Work out the finished part from the listing and answer in its coordinate system (mm). A direction names the side the tool comes from. Give positions to 0.01 mm unless a question says otherwise; leave off trailing zeros. Loops run counter-clockwise (first coordinate to the right, second up) from the corner with the lowest first, then second, coordinate; pieces in that order, holes last. Notation, with made-up numbers: (50.5, 44) - (90.5, 44) arc R20 cw to (90.5, 61) - close; hole circle Ø8 at (8, 26.5). An arc over 180 degrees is marked (long way). One line per question, with ' | ' between items.
from build123d import *

# Parameters (mm, degrees)
F0_R     = 1.7272
F0_R_2   = 2.15265
F0_R_3   = 9.525
F0_R_4   = 36.195
F1_DEPTH = 3.175
F2_R     = 4.7625


with BuildPart() as f1:
    # F0 (on Top) → F1 (new body)
    with BuildSketch(Plane.XY):
        with BuildLine():
            Line((-19.1686927371, 36.195), (-66.6623, 36.195))
            Line((-66.6623, 36.195), (-66.6623, -35.3695))
            Line((-66.6623, -35.3695), (-44.2988323935, -35.3695))
            Line((-44.2988323935, -35.3695), (-14.5929161967, -65.0754161967))
            ThreePointArc((-14.5929161967, -65.0754161967), (0, -71.12), (14.5929161967, -65.0754161967))
            Line((14.5929161967, -65.0754161967), (44.2988323935, -35.3695))
            Line((44.2988323935, -35.3695), (66.6623, -35.3695))
            Line((66.6623, -35.3695), (66.6623, 36.195))
            Line((66.6623, 36.195), (19.1686927371, 36.195))
            ThreePointArc((19.1686927371, 36.195), (0, 40.9575), (-19.1686927371, 36.195))
        make_face()
        with Locations((-11.7865861589, -62.2690861589)):
            Circle(F0_R, mode=Mode.SUBTRACT)
        with Locations((-61.8998, -30.607)):
            Circle(F0_R_2, mode=Mode.SUBTRACT)
        with Locations((-11.7865861589, -38.6959138411)):
            Circle(F0_R, mode=Mode.SUBTRACT)
        with Locations((11.7865861589, -62.2690861589)):
            Circle(F0_R, mode=Mode.SUBTRACT)
        with Locations((0, -50.4825)):
            Circle(F0_R_3, mode=Mode.SUBTRACT)
        with Locations((11.7865861589, -38.6959138411)):
            Circle(F0_R, mode=Mode.SUBTRACT)
        with Locations((61.8998, -30.607)):
            Circle(F0_R_2, mode=Mode.SUBTRACT)
        with Locations((-61.8998, 31.4325)):
            Circle(F0_R_2, mode=Mode.SUBTRACT)
        Circle(F0_R_4, mode=Mode.SUBTRACT)
        with Locations((61.8998, 31.4325)):
            Circle(F0_R_2, mode=Mode.SUBTRACT)
    extrude(amount=F1_DEPTH)

    # F2
    f2_edges = [f1.edges().sort_by_distance(p)[0] for p in [
        (66.6623, -35.3695, 1.5875),
        (-66.6623, -35.3695, 1.5875),
        (66.6623, 36.195, 1.5875),
        (-66.6623, 36.195, 1.5875),
    ]]
    fillet(f2_edges, radius=F2_R)


solid = f1.part
1. Flat-ended cylindrical pins translate along their axes: pin 1 (4 mm diameter, centred on x = 61.9, y = -30.61, fed in from +Z); pin 2 (1 mm diameter, centred on x = 55.5, z = 1, fed in from -Y); pin 3 (7 mm diameter, centred on x = 61.9, y = 31.43, fed in from +Z) (3 decimals); pin 4 (1.5 mm diameter, centred on y = -48.5, z = 2.5, fed in from +X). Find the tip coordinate at first contact, or state that the pin passes through.
Evaluation:
pin 1: through | pin 2: y = -35.37 | pin 3: z = 3.175 | pin 4: x = 31.92
2. Find section D-D on x = 21. Write down the section's boundary in (y, z) (3 decimals), then the cut area to 3 significant figures.
Evaluation:
outline: (-58.668, 0) - (-29.48, 0) - (-29.48, 3.175) - (-58.668, 3.175) - close; (29.48, 0) - (36.195, 0) - (36.195, 3.175) - (29.48, 3.175) - close | area: 114 mm2
3. Consider L1, parallel to X at y = -38.5, z = 1.9; L2, parallel to Y at x = 10.5, z = 1.55; L3, parallel to X at y = -62.5, z = 0.7. Determine where each line is inside the solid, lowest interval first.
Evaluation:
L1: -41.17 to -13.5, -10.07 to 10.07, 13.5 to 41.17 | L2: -68.25 to -63.42, -61.12 to -39.85, -37.54 to -34.64, 34.64 to 39.59 | L3: -17.17 to -13.5, -10.07 to 10.07, 13.5 to 17.17
4. Which of the six approach directions +Z, -Z, +X, -X, +Y, -Y give full straight-line access (tool end or side, diameter ignored) to faces 1 (the flat face through (53, -35.37, 2)), 2 (the cylindrical face through (0.279, 40.957, 1.565)), 3 (the flat face through (-40, 36.195, 2))?
Evaluation:
face 1: +Z, -Z, +X, -Y | face 2: +Z, -Z, +Y | face 3: +Z, -Z, -X, +Y
5. Find section C-C on z = 2.45. State how many separate pieces and enclosed holes the cut face has, then the cut area to 3 significant figures.
Evaluation:
separate pieces: 1 | enclosed holes: 10 | area: 7,020 mm2
6. Determine the mould class of faces 4 (the cylindrical face through (-12.011, -36.983, 1.565)), 5 (the cylindrical face through (-65.3, -33.94, 1.61)), 6 (the cylindrical face through (-65.23, 34.837, 1.61)) for opening direction Y: +Y half, -Y half, draft (parallel to the pull), parting line (faces both ways), or undercut.
Evaluation:
face 4: undercut | face 5: -Y half | face 6: +Y half
7. Find section A-A on y = 0. Write down the section's boundary in (x, z) (3 decimals).
Evaluation:
outline: (-66.662, 0) - (-36.195, 0) - (-36.195, 3.175) - (-66.662, 3.175) - close; (36.195, 0) - (66.662, 0) - (66.662, 3.175) - (36.195, 3.175) - close
8. Find section B-B on x = 0. Write down the section's boundary in (y, z) (1 decimal), then the cut area to 3 significant figures.
Evaluation:
outline: (-71.1, 0) - (-60, 0) - (-60, 3.2) - (-71.1, 3.2) - close; (-41, 0) - (-36.2, 0) - (-36.2, 3.2) - (-41, 3.2) - close; (36.2, 0) - (41, 0) - (41, 3.2) - (36.2, 3.2) - close | area: 65.5 mm2
